from build123d import *

# Parameters (mm, degrees)
F0_R     = 50
F0_R_2   = 23.297253
F1_DEPTH = 50
F2_R     = 23.297253
F3_DEPTH = 5
F4_R     = 12.970744
F4_R_2   = 5.052193
F5_DEPTH = 80


with BuildPart() as f1:
    # F0 (on Top) → F1 (new body)
    with BuildSketch(Plane.XY):
        with Locations((-12.402253, 3.797938)):
            Circle(F0_R)
        with Locations((-12.402253, 3.797938)):
            Circle(F0_R_2, mode=Mode.SUBTRACT)
    extrude(amount=F1_DEPTH)

    # F2 (on face) → F3 (join)
    with BuildSketch(Plane.XY.offset(50)):
        with Locations((-12.402253, 3.797938)):
            Circle(F2_R)
    extrude(amount=-F3_DEPTH)

    # F4 (on face) → F5 (join)
    with BuildSketch(Plane.XY.offset(50)):
        with Locations((-12.402253, 3.797938)):
            Circle(F4_R)
        with Locations((-12.402253, 3.797938)):
            Circle(F4_R_2, mode=Mode.SUBTRACT)
    extrude(amount=F5_DEPTH)


solid = f1.part
CAD build for the part. Positions are in the model's coordinates, mm. A direction names the side the tool comes from. Coordinates: 2 decimals unless noted, no trailing zeros. Loops run counter-clockwise (first coordinate to the right, second up) from the corner with the lowest first, then second, coordinate; pieces in that order, holes last. Notation, with made-up numbers: (13, -5) -> (71, -5) arc R18 cw to (71, 22) -> close; hole circle Ø5 at (23, 4). An arc over 180 degrees is marked (long way). One line per item, written item: value.
1. Slice it at C-C on z = 63.5. Write the cut outline in (x, y).
Answers:
outline: circle Ø25.94 at (-12.4, 3.8); hole circle Ø10.1 at (-12.4, 3.8)
2. Slice it at A-A on y = 24.5. Write the cut outline in (x, z), and give its area (3 significant figures).
Answers:
outline: (-57.92, 0) -> (-23.09, 0) -> (-23.09, 45) -> (-1.72, 45) -> (-1.72, 0) -> (33.11, 0) -> (33.11, 50) -> (-57.92, 50) -> close
area: 3,590 mm^2
3. Pull direction X, two halves, no side cores. Call faces 1 (the face through (-2, -7, 50)), 2 (the face through (-13, 4, 45)), 3 (the face through (33.785, -15.352, 24.65)): pulls with the +X half, pulls with the -X half, needs draft (parallel to the pull), parting line crosses it, or undercut.
Answers:
face 1: needs draft
face 2: undercut
face 3: parting line crosses it
4. Slice it at B-B on x = -9.5. Write the cut outline in (y, z), and give its area (3 significant figures).
Answers:
outline: (-46.12, 0) -> (-19.32, 0) -> (-19.32, 45) -> (26.91, 45) -> (26.91, 0) -> (53.71, 0) -> (53.71, 50) -> (16.44, 50) -> (16.44, 130) -> (7.93, 130) -> (7.93, 50) -> (-0.34, 50) -> (-0.34, 130) -> (-8.84, 130) -> (-8.84, 50) -> (-46.12, 50) -> close
area: 4,270 mm^2
5. Slice it at D-D on y = 1. Write the cut outline in (x, z).
Answers:
outline: (-62.32, 0) -> (-35.53, 0) -> (-35.53, 45) -> (10.73, 45) -> (10.73, 0) -> (37.52, 0) -> (37.52, 50) -> (0.26, 50) -> (0.26, 130) -> (-8.2, 130) -> (-8.2, 50) -> (-16.61, 50) -> (-16.61, 130) -> (-25.07, 130) -> (-25.07, 50) -> (-62.32, 50) -> close
6. Flat gauge pins, fed straight in: P1, Ø3, axis at x = 2, y = -17.5, coming from the +Z side; P2, Ø3, axis at y = 15, z = 103.5, coming from the -X side; P3, Ø6, axis at x = 14, z = 46.5, coming from the +Y side. Where does each tip first touch, or does it go through?
Answers:
P1: stops at z = 50
P2: stops at x = -21.01
P3: stops at y = 47.98
7. Which spindle directions (+Z, -Z, +X, -X, +Y, -Y) get a long thin tool onto all of the face, cutting with end or side? Do faces 4 (the face through (-30.89, -10.38, 22.18)), 5 (the face through (-7, 4, 130)), 6 (the face through (-13.497, -1.134, 89.44)). Say none if no direction does.
Answers:
face 4: -Z
face 5: +Z, +X, -X, +Y, -Y
face 6: +Z
8. Drill centre lines: line 1 (Y direction, x = -10, z = 15.5); line 2 (Y direction, x = -7.5, z = 36); line 3 (Z direction, x = -15, y = -20). Where is each one in solid material? Low to high. Write a range as [from, to].
Answers:
line 1: y = [-46.14, -19.38], [26.97, 53.74]
line 2: y = [-45.96, -18.98], [26.57, 53.56]
line 3: z = [0, 50]
